Autodesk Inventor part; units mm, degrees
ref_plane "YZ Plane" through (0, 0, 0) normal (1, 0, 0) x (0, 1, 0)
ref_plane "XZ Plane" through (0, 0, 0) normal (0, 1, 0) x (-1, 0, 0)
ref_plane "XY Plane" through (0, 0, 0) normal (0, 0, 1) x (1, 0, 0)
sketch "Sketch1" plane through (0, 0, 0) normal (0, 1, 0) x (-1, 0, 0)
  line L0 (0, 0) -> (203.2, 0)
  line L1 (203.2, 0) -> (203.2, -254)
  line L2 (203.2, -254) -> (0, -254)
  line L3 (0, -254) -> (0, 0)
  line L4 (203.2, -127) -> (0, -127)
  line L5 (101.6, -254) -> (101.6, 0)
  circle A0 centre (101.6, -127) radius 69.85
  point P0 (171.45, -127)
  point P1 (31.75, -127)
  point P2 (101.6, -57.15)
  point P3 (101.6, -196.85)
  dimension "d0" = 203.2
  dimension "d1" = 254
  dimension "d2" = 139.7
extrude "Extrusion1" add sketch "Sketch1" along normal blind 3.175 contours L0 L5 A0 L4 L3 | L4 A0 L5 L2 L3
properties part number "1 Bottom Frame Base 1"
Check sheet for the modelled part. Datum: model origin and axes. Units: mm. Round coordinates to 2 decimals unless told otherwise and drop trailing zeros. Loops run counter-clockwise (first coordinate to the right, second up) from the corner with the lowest first, then second, coordinate; pieces in that order, holes last.
1. Sectioned sample at D-D on x = -94. Record the boundary of the cut face in (y, z) (3 decimals).
2. Sectioned sample at C-C on z = -127. Record the boundary of the cut face in (x, y) (3 decimals).
3. Sectioned sample at B-B on y = 2.15. Record the boundary of the cut face in (x, z), and give its area (3 significant figures).
4. Sectioned sample at A-A on x = -58. Record the boundary of the cut face in (y, z) (3 decimals), and give its area (3 significant figures).
5. Scan lines: probe 1 along Z at (x, y) = (-78, 2); probe 2 along Z at (x, y) = (-37.5, 3); probe 3 along X at (y, z) = (2.7, -85.5). Record each from-to range of solid material in increasing order.
6. Mould release check, pull along Z, two halves, no side actions. Record for faces 1 (the cylindrical face through (-31.767, 1.565, -128.536)), 2 (the flat face through (-28, 0, -125)): released by +Z, released by -Z, zero draft, split by the parting line, or undercut.
7. Gauge pin test, flat end, axial feed: pin 1 Ø4 at (x, z) = (-17, -204.5) entering from -Y. Record the tip position at first contact, or that the pin passes through.
Recorded:
1. outline: (0, -254) - (3.175, -254) - (3.175, -196.435) - (0, -196.435) - close; (0, -57.565) - (3.175, -57.565) - (3.175, 0) - (0, 0) - close
2. outline: (-31.75, 0) - (0, 0) - (0, 3.175) - (-31.75, 3.175) - close
3. outline: (-101.6, -254) - (0, -254) - (0, 0) - (-101.6, 0) - (-101.6, -57.15) arc R69.85 cw to (-101.6, -196.85) - close
3. area: 18,100 mm2
4. outline: (0, -254) - (3.175, -254) - (3.175, -181.572) - (0, -181.572) - close; (0, -72.428) - (3.175, -72.428) - (3.175, 0) - (0, 0) - close
4. area: 460 mm2
5. probe 1: z = -254 to -192.74, -61.26 to 0
5. probe 2: z = -254 to -154.75, -99.25 to 0
5. probe 3: x = -45.41 to 0
6. face 1: undercut
6. face 2: zero draft
7. pin 1: stops at y = 0
